Autodesk Inventor part; units mm, degrees
ref_plane "bf_1_XY" through (0, 0, 0) normal (0, 0, 1) x (1, 0, 0)
ref_plane "bf_1_YZ" through (0, 0, 0) normal (1, 0, 0) x (0, 1, 0)
ref_plane "bf_1_ZX" through (0, 0, 0) normal (0, 1, 0) x (0, 0, 1)
sketch "Sketch_1" plane through (0, 0, 0) normal (0, 0, 1) x (1, 0, 0)
  line L0 (-40, -45) -> (-40, 10)
  line L1 (-40, 10) -> (-20.5, 10)
  line L2 (-20.5, 10) -> (-20.5, 20)
  line L3 (-20.5, 20) -> (20.5, 20)
  line L4 (20.5, 20) -> (20.5, 10)
  line L5 (20.5, 10) -> (40, 10)
  line L6 (40, 10) -> (40, -45)
  line L7 (40, -45) -> (-40, -45)
  line L8 (-40, -45) -> (-40, -25)
  dimension "d24" = 55
  dimension "d25" = 19.5
  dimension "d26" = 10
  dimension "d27" = 41
  dimension "d28" = 10
  dimension "d29" = 19.5
  dimension "d30" = 55
  dimension "d31" = 20
extrude "Extrusion1" add sketch "Sketch_1" against normal blind 20
ref_plane "bf_1_XY" through (0, 0, 0) normal (0, 0, 1) x (1, 0, 0)
ref_plane "bf_1_YZ" through (0, 0, 0) normal (1, 0, 0) x (0, 1, 0)
ref_plane "bf_1_ZX" through (0, 0, 0) normal (0, 1, 0) x (0, 0, 1)
ref_plane "bf_2x_XY" through (0, 0, -10) normal (0, 0, 1) x (1, 0, 0)
ref_plane "bf_2x_YZ" through (0, 0, -10) normal (1, 0, 0) x (0, 1, 0)
ref_plane "bf_2x_ZX" through (0, 0, -10) normal (0, 1, 0) x (0, 0, 1)
sketch "Sketch6" plane through (20.5, 10, 0) normal (0, 1, 0) x (1, 0, 0)
  line L0 (-41, 0) -> (0, 0)
  line L1 (19.5, 0) -> (19.5, 20)
  line L2 (19.5, 10) -> (9.5, 10)
  line L3 (-60.5, 0) -> (-60.5, 20)
  line L4 (-60.5, 10) -> (-50.5, 10)
  point P0 (-20.5, 0)
  dimension "d32" = 10
  dimension "d40" = 10
hole "Hole4" at (30, 10, -10) at (-30, 10, -10) direction (0, -1, 0) diameter 10.5 end through all counterbore diameter 17 counterbore depth 12
sketch "Sketch7" plane through (0, 0, 0) normal (0, 0, 1) x (1, 0, 0)
  circle A0 centre (0, 0) radius 16
  dimension "d42" = 32
extrude "Extrusion2" cut sketch "Sketch7" against normal up to surface (20 mm away)
properties part number "BF 15 Part1"
Design review of the part built by this model. Coordinates are the model's own, in mm. A direction names the side the tool comes from. Round coordinates to 2 decimals unless told otherwise and drop trailing zeros. Order: outer loops, then holes, each group sorted by start corner. A loop starts at its lowest first (then second) coordinate and runs counter-clockwise, first axis right, second up. Notation, with made-up numbers: M 23.5,-32 L 79.5,-32 A24 cw 79.5,-19 Z; hole C 23,72 d11. An arc over 180 degrees is marked long. Answer as CSV lines item,"result". Start each with the question number.
1) Add section B-B (y = 0). Give the boundary of the cut face in (x, z).
2) The part is to be moulded in two halves that separate along Z. For faces 1 (the face through (-1, -19, -20)), 2 (the face through (39, 10, -10)), 3 (the face through (34, -2, -14)), say which applies: +Z half, -Z half, draft (parallel to the pull), parting line (faces both ways), or undercut.
3) Wall thickness on line 1 along X through (y, z) = (-21, -10); line 2 along Z through (x, y) = (-30, 6); line 3 along X through (y, z) = (-17.5, -8.25): over which ranges is each line inside the solid? List them lowest first. Write a range as [from, to].
4) Add section A-A (z = -10). Give the boundary of the cut face in (x, y), then the cut area to 3 significant figures.
5) Add section C-C (x = 0). Give the boundary of the cut face in (y, z), then the cut area to 3 significant figures.
6) Add section D-D (y = 8). Give the boundary of the cut face in (x, z), then the cut area to 3 significant figures.
7) For pin 1 Ø12 at (x, z) = (-30, -10) entering from +Y; pin 2 Ø8 at (y, z) = (16, -12.5) entering from +X; pin 3 Ø5 at (y, z) = (17, -6.5) entering from -X, all flat-tipped, find the tip position at first contact; note any pin that passes through.
8) Tool access review of faces 4 (the face through (-40, -18, -10)), 5 (the face through (-39, 10, -10)), 6 (the face through (-26, -2, -14)), 7 (the face through (20.5, 15, -10)): name each direction out of +Z, -Z, +X, -X, +Y, -Y from which nothing blocks a thin tool from reaching the whole face with its end or side.
Resolved:
1,outline,"M -40,-20 L -16,-20 L -16,0 L -40,0 Z; M 16,-20 L 40,-20 L 40,0 L 16,0 Z; hole C -30,-10 d17; hole C 30,-10 d17"
2,face 1,"-Z half"
2,face 2,"draft"
2,face 3,"undercut"
3,line 1,"[-40, -35.25], [-24.75, 24.75], [35.25, 40]"
3,line 2,"[-20, -18.5], [-1.5, 0]"
3,line 3,"[-40, -34.95], [-25.05, 25.05], [34.95, 40]"
4,outline,"M -40,-45 L -35.25,-45 L -35.25,-2 L -38.5,-2 L -38.5,10 L -40,10 Z; M -24.75,-45 L 24.75,-45 L 24.75,-2 L 21.5,-2 L 21.5,10 L 20.5,10 L 20.5,20 L -20.5,20 L -20.5,10 L -21.5,10 L -21.5,-2 L -24.75,-2 Z; M 35.25,-45 L 40,-45 L 40,10 L 38.5,10 L 38.5,-2 L 35.25,-2 Z; hole C 0,0 d32"
4,area,"2,690 mm^2"
5,outline,"M -45,-20 L -16,-20 L -16,0 L -45,0 Z; M 16,-20 L 20,-20 L 20,0 L 16,0 Z"
5,area,"660 mm^2"
6,outline,"M -40,-20 L -13.86,-20 L -13.86,0 L -40,0 Z; M 13.86,-20 L 40,-20 L 40,0 L 13.86,0 Z; hole C -30,-10 d17; hole C 30,-10 d17"
6,area,"592 mm^2"
7,pin 1,"y = -2"
7,pin 2,"x = 20.5"
7,pin 3,"x = -20.5"
8,face 4,"+Z, -Z, -X, +Y, -Y"
8,face 5,"+Z, -Z, -X, +Y"
8,face 6,"+Y"
8,face 7,"+Z, -Z, +X, +Y"
